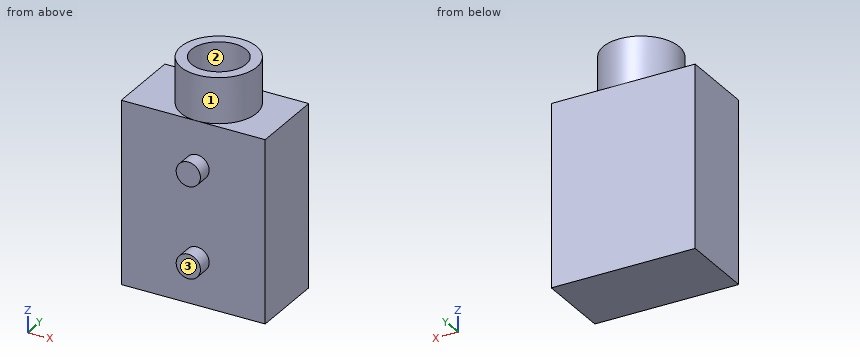
from build123d import *

# Parameters (mm, degrees)
SKETCH1_W           = 9.5
SKETCH1_H           = 12
BOSS_EXTRUDE1_DEPTH = 5
SKETCH2_R           = 2.5
SKETCH2_R_2         = 1.8
BOSS_EXTRUDE2_DEPTH = 3
SKETCH3_R           = 0.8
BOSS_EXTRUDE3_DEPTH = 1


with BuildPart() as part:
    # Sketch1 → Boss-Extrude1 (new body)
    with BuildSketch(Plane(origin=(0, 0, 0), x_dir=(1, 0, 0), z_dir=(0, 1, 0))):
        with Locations((4.75, 6)):
            Rectangle(SKETCH1_W, SKETCH1_H)
    extrude(amount=BOSS_EXTRUDE1_DEPTH)

    # Sketch2 → Boss-Extrude2 (add)
    with BuildSketch(Plane.XY):
        with Locations(Location((5, 2.5, 0), (0, 0, 270))):
            Circle(SKETCH2_R)
        with Locations((5, 2.5)):
            Circle(SKETCH2_R_2, mode=Mode.SUBTRACT)
    extrude(amount=BOSS_EXTRUDE2_DEPTH)

    # Sketch3 → Boss-Extrude3 (add)
    with BuildSketch(Plane.XZ):
        with Locations(Location((5, -3, 0), (0, 0, 270))):
            Circle(SKETCH3_R)
        with Locations(Location((5, -9, 0), (0, 0, 270))):
            Circle(SKETCH3_R)
    extrude(amount=BOSS_EXTRUDE3_DEPTH)


solid = part.part
Model file for the job. Use its own axes, mm. Face numbers are marked on the shaded views. Give positions to 0.01 mm unless a question says otherwise; leave off trailing zeros. Order: outer loops, then holes, each group sorted by start corner. A loop starts at its lowest first (then second) coordinate and runs counter-clockwise, first axis right, second up. Notation, with made-up numbers: (41, -8) - (88, -8) arc R28 cw to (88, 20) - close; hole circle Ø7 at (-19.5, 82.5). An arc over 180 degrees is marked (long way). One line per item, written item: value.
Item 1: Two-plate mould, pull along X, no slides. Class the marked faces 1, 2 and 3: released by +X, released by -X, zero draft, split by the parting line, or undercut.
Response values:
face 1: split by the parting line
face 2: undercut
face 3: zero draft
Item 2: Slice it at B-B (y = 0.5). List the corners of the cut face in (x, z), then the cut area to 3 significant figures.
Response values:
outline: (0, -12) - (9.5, -12) - (9.5, 0) - (6.5, 0) - (6.5, 3) - (3.5, 3) - (3.5, 0) - (0, 0) - close
area: 123 mm2
Item 3: Slice it at C-C (y = -0.6). List the corners of the cut face in (x, z).
Response values:
outline: circle Ø1.6 at (5, -9); circle Ø1.6 at (5, -3)
Item 4: Wall check: line 1 (Y direction, x = 5, z = 1.6); line 2 (Y direction, x = 6.25, z = -7); line 3 (Z direction, x = 2, y = 2.5). Give the ranges that are in metal, low to high.
Response values:
line 1: 0 to 0.7, 4.3 to 5
line 2: 0 to 5
line 3: -12 to 0
Item 5: Slice it at A-A (x = 7). List the corners of the cut face in (y, z).
Response values:
outline: (0, -12) - (5, -12) - (5, 0) - (4, 0) - (4, 3) - (1, 3) - (1, 0) - (0, 0) - close
Item 6: Slice it at D-D (z = 1.5). List the corners of the cut face in (x, y), then the cut area to 3 significant figures.
Response values:
outline: circle Ø5 at (5, 2.5); hole circle Ø3.6 at (5, 2.5)
area: 9.46 mm2
